```python
from build123d import *

# Parameters (mm, degrees)
SKETCH1_W                                      = 100
SKETCH1_H                                      = 84
BOSS_EXTRUDE1_DEPTH                            = 8
CBORE_FOR_2_SOCKET_HEAD_CAP_SCREW1_D           = 2.4384
CBORE_FOR_2_SOCKET_HEAD_CAP_SCREW1_DEPTH       = 12.27
CBORE_FOR_2_SOCKET_HEAD_CAP_SCREW1_CBORE_D     = 4.7625
CBORE_FOR_2_SOCKET_HEAD_CAP_SCREW1_CBORE_DEPTH = 2.1844
CBORE_FOR_2_SOCKET_HEAD_CAP_SCREW1_TIP         = 0.732569267
CBORE_FOR_2_SOCKET_HEAD_CAP_SCREW2_D           = 2.4384
CBORE_FOR_2_SOCKET_HEAD_CAP_SCREW2_DEPTH       = 12.27
CBORE_FOR_2_SOCKET_HEAD_CAP_SCREW2_CBORE_D     = 4.7625
CBORE_FOR_2_SOCKET_HEAD_CAP_SCREW2_CBORE_DEPTH = 2.1844
CBORE_FOR_2_SOCKET_HEAD_CAP_SCREW2_TIP         = 0.732569267
F_2_56_TAPPED_HOLE1_D                          = 1.778
F_2_56_TAPPED_HOLE1_DEPTH                      = 12
F_2_56_TAPPED_HOLE1_TIP                        = 0.53416509
SKETCH12_W                                     = 35
SKETCH12_H                                     = 60
CUT_EXTRUDE3_DEPTH                             = 3
FILLET1_R                                      = 2
FILLET2_R                                      = 2
FILLET3_R                                      = 2
FILLET4_R                                      = 2
SKETCH17_W                                     = 11
SKETCH17_H                                     = 19.5
CUT_EXTRUDE4_DEPTH                             = 8
SKETCH16_W                                     = 11
SKETCH16_H                                     = 19.5
CUT_EXTRUDE5_DEPTH                             = 8
FILLET5_R                                      = 2
FILLET6_R                                      = 2
FILLET7_R                                      = 2
FILLET8_R                                      = 2
F_4_40_TAPPED_HOLE1_D                          = 2.2606
SKETCH21_R                                     = 2
CUT_EXTRUDE6_DEPTH                             = 8
FILLET9_R                                      = 3


with BuildPart() as part:
    # Sketch1 → Boss-Extrude1 (new body)
    with BuildSketch(Plane.XY):
        Rectangle(SKETCH1_W, SKETCH1_H)
    extrude(amount=BOSS_EXTRUDE1_DEPTH)

    # CBORE for #2 Socket Head Cap Screw1
    with Locations(Plane(origin=(-32, -39, 8), x_dir=(1, 0, 0), z_dir=(0, 0, 1))):
        with Locations((0, 0), (64, 0)):
            CounterBoreHole(CBORE_FOR_2_SOCKET_HEAD_CAP_SCREW1_D / 2, CBORE_FOR_2_SOCKET_HEAD_CAP_SCREW1_CBORE_D / 2, CBORE_FOR_2_SOCKET_HEAD_CAP_SCREW1_CBORE_DEPTH, depth=CBORE_FOR_2_SOCKET_HEAD_CAP_SCREW1_DEPTH)
            with Locations((0, 0, -(CBORE_FOR_2_SOCKET_HEAD_CAP_SCREW1_DEPTH + CBORE_FOR_2_SOCKET_HEAD_CAP_SCREW1_TIP / 2))):  # 118° drill point
                Cone(0, CBORE_FOR_2_SOCKET_HEAD_CAP_SCREW1_D / 2, CBORE_FOR_2_SOCKET_HEAD_CAP_SCREW1_TIP, mode=Mode.SUBTRACT)

    # CBORE for #2 Socket Head Cap Screw2
    with Locations(Plane(origin=(-46, 0, 8), x_dir=(1, 0, 0), z_dir=(0, 0, 1))):
        with Locations((0, 0), (92, 0)):
            CounterBoreHole(CBORE_FOR_2_SOCKET_HEAD_CAP_SCREW2_D / 2, CBORE_FOR_2_SOCKET_HEAD_CAP_SCREW2_CBORE_D / 2, CBORE_FOR_2_SOCKET_HEAD_CAP_SCREW2_CBORE_DEPTH, depth=CBORE_FOR_2_SOCKET_HEAD_CAP_SCREW2_DEPTH)
            with Locations((0, 0, -(CBORE_FOR_2_SOCKET_HEAD_CAP_SCREW2_DEPTH + CBORE_FOR_2_SOCKET_HEAD_CAP_SCREW2_TIP / 2))):  # 118° drill point
                Cone(0, CBORE_FOR_2_SOCKET_HEAD_CAP_SCREW2_D / 2, CBORE_FOR_2_SOCKET_HEAD_CAP_SCREW2_TIP, mode=Mode.SUBTRACT)

    # #2-56 Tapped Hole1
    with Locations(Plane(origin=(-32, 42, 4), x_dir=(0, 0, 1), z_dir=(0, 1, 0))):
        with Locations((0, 0), (0, 64)):
            Hole(F_2_56_TAPPED_HOLE1_D / 2, depth=F_2_56_TAPPED_HOLE1_DEPTH)
            with Locations((0, 0, -(F_2_56_TAPPED_HOLE1_DEPTH + F_2_56_TAPPED_HOLE1_TIP / 2))):  # 118° drill point
                Cone(0, F_2_56_TAPPED_HOLE1_D / 2, F_2_56_TAPPED_HOLE1_TIP, mode=Mode.SUBTRACT)

    # Sketch12 → Cut-Extrude3 (cut)
    with BuildSketch(Plane(origin=(0, 0, 0), x_dir=(-1, 0, 0), z_dir=(0, 0, -1))):
        with Locations((24.5, 0)):
            Rectangle(SKETCH12_W, SKETCH12_H)
    extrude(amount=-CUT_EXTRUDE3_DEPTH, mode=Mode.SUBTRACT)

    # Fillet1
    fillet1_edges = [part.edges().sort_by_distance(p)[0] for p in [
        (-7, 30, 1.5),
    ]]
    fillet(fillet1_edges, radius=FILLET1_R)

    # Fillet2
    fillet2_edges = [part.edges().sort_by_distance(p)[0] for p in [
        (-42, 30, 1.5),
    ]]
    fillet(fillet2_edges, radius=FILLET2_R)

    # Fillet3
    fillet3_edges = [part.edges().sort_by_distance(p)[0] for p in [
        (-42, -30, 1.5),
    ]]
    fillet(fillet3_edges, radius=FILLET3_R)

    # Fillet4
    fillet4_edges = [part.edges().sort_by_distance(p)[0] for p in [
        (-7, -30, 1.5),
    ]]
    fillet(fillet4_edges, radius=FILLET4_R)

    # Sketch17 → Cut-Extrude4 (cut)
    with BuildSketch(Plane(origin=(0, 0, 3), x_dir=(-1, 0, 0), z_dir=(0, 0, -1))):
        with Locations((35, 0)):
            Rectangle(SKETCH17_W, SKETCH17_H)
    extrude(amount=-CUT_EXTRUDE4_DEPTH, mode=Mode.SUBTRACT)

    # Sketch16 → Cut-Extrude5 (cut)
    with BuildSketch(Plane(origin=(0, 0, 3), x_dir=(-1, 0, 0), z_dir=(0, 0, -1))):
        with Locations((14, 0)):
            Rectangle(SKETCH16_W, SKETCH16_H)
    extrude(amount=-CUT_EXTRUDE5_DEPTH, mode=Mode.SUBTRACT)

    # Fillet5
    fillet5_edges = [part.edges().sort_by_distance(p)[0] for p in [
        (-40.5, 9.75, 5.5),
        (-19.5, 9.75, 5.5),
    ]]
    fillet(fillet5_edges, radius=FILLET5_R)

    # Fillet6
    fillet6_edges = [part.edges().sort_by_distance(p)[0] for p in [
        (-29.5, 9.75, 5.5),
        (-8.5, 9.75, 5.5),
    ]]
    fillet(fillet6_edges, radius=FILLET6_R)

    # Fillet7
    fillet7_edges = [part.edges().sort_by_distance(p)[0] for p in [
        (-29.5, -9.75, 5.5),
        (-8.5, -9.75, 5.5),
    ]]
    fillet(fillet7_edges, radius=FILLET7_R)

    # Fillet8
    fillet8_edges = [part.edges().sort_by_distance(p)[0] for p in [
        (-40.5, -9.75, 5.5),
        (-19.5, -9.75, 5.5),
    ]]
    fillet(fillet8_edges, radius=FILLET8_R)

    # #4-40 Tapped Hole1 (through all)
    with Locations(Plane(origin=(-35, 12.5, 8), x_dir=(1, 0, 0), z_dir=(0, 0, 1))):
        with Locations((0, 0), (0, -25), (21, -25), (21, 0)):
            Hole(F_4_40_TAPPED_HOLE1_D / 2)

    # Sketch21 → Cut-Extrude6 (cut)
    with BuildSketch(Plane(origin=(0, 0, 3), x_dir=(-1, 0, 0), z_dir=(0, 0, -1))):
        with Locations((24.5, 25)):
            Circle(SKETCH21_R)
    extrude(amount=-CUT_EXTRUDE6_DEPTH, mode=Mode.SUBTRACT)

    # Fillet9
    # the kernel refuses this fillet: 3 mm, written as the material it takes off along each edge
    with BuildSketch(Plane(origin=(-50, -49.5, 8), x_dir=(1, 0, 0), z_dir=(0, 1, 0)), Plane(origin=(50, 49.5, 8), x_dir=(-1, 0, 0), z_dir=(0, -1, 0))) as fillet9_piece_1:
        with BuildLine():
            CenterArc((FILLET9_R, FILLET9_R), FILLET9_R, 180, 90)
            Line((0, FILLET9_R), (0, 0))
            Line((0, 0), (FILLET9_R, 0))
        make_face()
    extrude(amount=99, mode=Mode.SUBTRACT)


solid = part.part
```
Geometry check sheet. Reference: the model listing, model coordinates, mm. A direction names the side the tool comes from. Give positions to 0.01 mm unless a question says otherwise; leave off trailing zeros. Order: outer loops, then holes, each group sorted by start corner. A loop starts at its lowest first (then second) coordinate and runs counter-clockwise, first axis right, second up. Notation, with made-up numbers: (42.25, 26.25) - (79.25, 26.25) arc R12 cw to (79.25, 33.25) - close; hole circle Ø4 at (-6.5, -35.5). An arc over 180 degrees is marked (long way). Answer in a Markdown table with one row per item. Add a question column.
Q1. Gauge pin test, flat ends, axial feed: pin 1 (3 mm diameter, centred on y = -13, z = 7, fed in from +X); pin 2 (3.5 mm diameter, centred on x = -35, y = 12.5, fed in from +Z); pin 3 (3 mm diameter, centred on x = -32, y = -39, fed in from +Z). Record the tip position at first contact, or that the pin passes through.
Q2. Cross-section at D-D, the plane y = 19.5. Enter the section's corners in (x, z), then the cut area to 3 significant figures.
Q3. Cross-section at A-A, the plane x = -14. Enter the section's corners in (y, z), then the cut area to 3 significant figures.
Q4. Cross-section at C-C, the plane z = 1.25. Enter the section's corners in (x, y).
Q5. Material ranges on probe 1 along Y at (x, z) = (-35, 4.2); probe 2 along Y at (x, z) = (-32, 2.9); probe 3 along Y at (x, z) = (-32, 6.8), recorded low to high. Write a range as from..to.
Q6. Mould release check, pull along X, two halves, no side actions. Record for faces 1 (the cylindrical face through (-49.14, -0.59, 7.1)), 2 (the cylindrical face through (-12.87, -12.45, 5.47)), 3 (the flat face through (-1, 42, 4)): pulls with the +X half, pulls with the -X half, needs draft (parallel to the pull), parting line crosses it, or undercut.
Q7. Tool access check on faces 4 (the cylindrical face through (-18.9, -9.18, 5.54)), 5 (the flat face through (-33, -38, 5.816)), 6 (the cylindrical face through (-7.6, -29.43, 1.52)), 7 (the flat face through (-1, -42, 4)), 8 (the flat face through (10, 1, 0)). Record the directions out of +Z, -Z, +X, -X, +Y, -Y that give a thin tool (end or side, any length) a straight path to the whole face; none if there is none.
Q8. Cross-section at B-B, the plane y = -39. Enter the section's corners in (x, z).
Check values:
| question | item | result |
|---|---|---|
| 1 | pin 1 | stops at x = 49.96 |
| 1 | pin 2 | stops at z = 8 |
| 1 | pin 3 | stops at z = 5.82 |
| 2 | outline | (-50, 0) - (-42, 0) - (-42, 3) - (-7, 3) - (-7, 0) - (50, 0) - (50, 5) arc R3 ccw to (47, 8) - (-47, 8) arc R3 ccw to (-50, 5) - close |
| 2 | area | 691 mm^2 |
| 3 | outline | (-42, 0) - (-30, 0) - (-30, 3) - (-13.63, 3) - (-13.63, 8) - (-42, 8) - close; (-11.37, 3) - (-9.75, 3) - (-9.75, 8) - (-11.37, 8) - close; (9.75, 3) - (11.37, 3) - (11.37, 8) - (9.75, 8) - close; (13.63, 3) - (30, 3) - (30, 0) - (42, 0) - (42, 8) - (13.63, 8) - close |
| 3 | area | 372 mm^2 |
| 4 | outline | (-50, -42) - (50, -42) - (50, 42) - (-50, 42) - close; hole circle Ø2.44 at (-46, 0); hole (-42, -28) arc R2 ccw to (-40, -30) - (-9, -30) arc R2 ccw to (-7, -28) - (-7, 28) arc R2 ccw to (-9, 30) - (-40, 30) arc R2 ccw to (-42, 28) - close; hole circle Ø2.44 at (-32, -39); hole circle Ø2.44 at (32, -39); hole circle Ø2.44 at (46, 0) |
| 5 | probe 1 | y = -42..-13.63, -11.37..-9.75, 9.75..11.37, 13.63..42 |
| 5 | probe 2 | y = -42..-40.22, -37.78..-30, 30..42 |
| 5 | probe 3 | y = -42..-41.38, -36.62..-9.75, 9.75..42 |
| 6 | face 1 | pulls with the -X half |
| 6 | face 2 | undercut |
| 6 | face 3 | needs draft |
| 7 | face 4 | +Z, -Z |
| 7 | face 5 | +Z |
| 7 | face 6 | -Z |
| 7 | face 7 | +Z, -Z, +X, -X, -Y |
| 7 | face 8 | -Z, +X, -X, +Y, -Y |
| 8 | outline | (-50, 0) - (-33.22, 0) - (-33.22, 5.82) - (-34.38, 5.82) - (-34.38, 8) - (-47, 8) arc R3 ccw to (-50, 5) - close; (-30.78, 0) - (30.78, 0) - (30.78, 5.82) - (29.62, 5.82) - (29.62, 8) - (-29.62, 8) - (-29.62, 5.82) - (-30.78, 5.82) - close; (33.22, 0) - (50, 0) - (50, 5) arc R3 ccw to (47, 8) - (34.38, 8) - (34.38, 5.82) - (33.22, 5.82) - close |
